Autodesk Inventor part; units mm, degrees
ref_plane "YZ Plane" through (0, 0, 0) normal (1, 0, 0) x (0, 1, 0)
ref_plane "XZ Plane" through (0, 0, 0) normal (0, 1, 0) x (-1, 0, 0)
ref_plane "XY Plane" through (0, 0, 0) normal (0, 0, 1) x (1, 0, 0)
sketch "Sketch2" plane through (0, 0, 0) normal (0, 0, 1) x (1, 0, 0)
  circle A0 centre (0, 0) radius 30.099
  circle A1 centre (0, 63.5) radius 3.175
  circle A2 centre (-54.9926, -31.75) radius 3.175
  circle A3 centre (54.9926, -31.75) radius 3.175
  line L0 (0, 69.85) -> (60.4919, -34.925) construction
  line L1 (60.4919, -34.925) -> (-60.4919, -34.925) construction
  line L2 (-60.4919, -34.925) -> (0, 69.85) construction
  line L3 (0, 95.25) -> (82.4889, -47.625)
  line L4 (82.4889, -47.625) -> (-82.4889, -47.625)
  line L5 (-82.4889, -47.625) -> (0, 95.25)
  dimension "d0" = 60.198
  dimension "d1" = 6.35
  dimension "d2" = 63.5
  dimension "d5" = 360
  dimension "d8" = 12.7
  dimension "d9" = 12.7
  dimension "d10" = 12.7
extrude "Extrusion1" add sketch "Sketch2" along normal blind 3.175
fillet "Fillet1" radius 19.05 3 edges at (0, 95.25, 1.5875) (-82.4889, -47.625, 1.5875) (82.4889, -47.625, 1.5875)
properties part number "Triangle-PVC-hole"
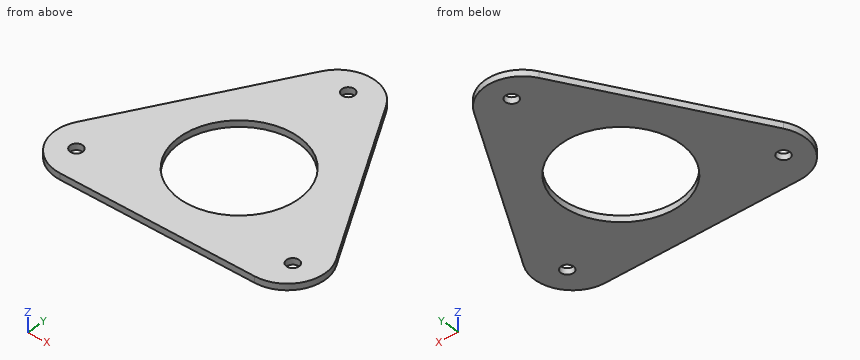
The model under review builds one solid part; all positions refer to its coordinate system, in mm. Coordinates: 2 decimals unless noted, no trailing zeros. Write each loop counter-clockwise with the first axis right and the second up, starting at its lowest first coordinate (ties: lowest second). Pieces come first, ordered by that corner, then holes.
1) We need section B-B on z = 2. State the section outline as (x, y) points (3 decimals).
2) We need section D-D on x = -14. State the section outline as (y, z) points (3 decimals), then the cut area to 3 significant figures.
3) Clearance check with flat-ended pins moving along their axes: pin 1 Ø7.5 at (x, y) = (-54.99, -31.75) entering from +Z (3 decimals); pin 2 Ø1.5 at (x, z) = (-53.5, 2) entering from -Y. State where each tip first meets the part, or that it passes through.
4) We need section A-A on x = 0. State the section outline as (y, z) points (3 decimals).
5) We need section C-C on y = 0. State the section outline as (x, z) points (3 decimals), then the cut area to 3 significant figures.
6) To check wall thickness, follow probe 1 along Y at (x, z) = (0, 1.15) (3 decimals); probe 2 along X at (y, z) = (-32.5, 1.5); probe 3 along X at (y, z) = (13, 2.4). State the ranges of each line that lie inside material, in increasing order.
Answer list:
1. outline: (-65.991, -19.05) arc R19.05 ccw to (-49.493, -47.625) - (49.493, -47.625) arc R19.05 ccw to (65.991, -19.05) - (16.498, 66.675) arc R19.05 ccw to (-16.498, 66.675) - close; hole circle Ø6.35 at (-54.993, -31.75); hole circle Ø60.198 at (0, 0); hole circle Ø6.35 at (0, 63.5); hole circle Ø6.35 at (54.993, -31.75)
2. outline: (-47.625, 0) - (-26.645, 0) - (-26.645, 3.175) - (-47.625, 3.175) - close; (26.645, 0) - (70.069, 0) - (70.069, 3.175) - (26.645, 3.175) - close
2. area: 204 mm2
3. pin 1: stops at z = 3.175
3. pin 2: stops at y = -47.34
4. outline: (-47.625, 0) - (-30.099, 0) - (-30.099, 3.175) - (-47.625, 3.175) - close; (30.099, 0) - (60.325, 0) - (60.325, 3.175) - (30.099, 3.175) - close; (66.675, 0) - (76.2, 0) - (76.2, 3.175) - (66.675, 3.175) - close
5. outline: (-54.993, 0) - (-30.099, 0) - (-30.099, 3.175) - (-54.993, 3.175) - close; (30.099, 0) - (54.993, 0) - (54.993, 3.175) - (30.099, 3.175) - close
5. area: 158 mm2
6. probe 1: y = -47.625 to -30.099, 30.099 to 60.325, 66.675 to 76.2
6. probe 2: x = -68.13 to -58.08, -51.91 to 51.91, 58.08 to 68.13
6. probe 3: x = -47.49 to -27.15, 27.15 to 47.49
